Autodesk Inventor part; units mm, degrees
ref_plane "YZ Plane" through (0, 0, 0) normal (1, 0, 0) x (0, 1, 0)
ref_plane "XZ Plane" through (0, 0, 0) normal (0, 1, 0) x (-1, 0, 0)
ref_plane "XY Plane" through (0, 0, 0) normal (0, 0, 1) x (1, 0, 0)
sketch "Эскиз1" plane through (0, 0, 0) normal (0, 0, 1) x (1, 0, 0)
  line L0 (0, 0) -> (10, 0)
  line L1 (10, 0) -> (10, 10)
  line L2 (10, 10) -> (0, 10)
  line L3 (0, 10) -> (0, 0)
  dimension "d5" = 10
  dimension "d6" = 10
sketch "Эскиз2" plane through (0, 0, 0) normal (0, 1, 0) x (-1, 0, 0)
  line L0 (0, 0) -> (0, 200)
  line L1 (-50, 250) -> (-250, 250)
  arc A0 (0, 200) -> (-50, 250) centre (-50, 200) ccw
  point P0 (0, 250)
  dimension "d3" = 250
  dimension "d4" = 250
  dimension "d7" = 50
sweep "Сдвиг1" add profiles "Эскиз1" path "Эскиз2"
properties part number "4"
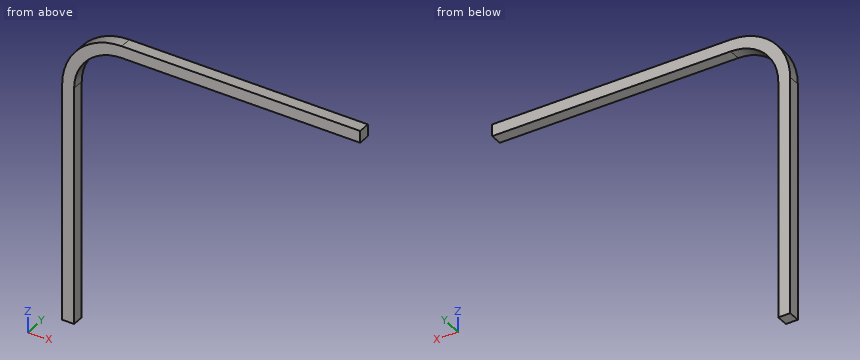
Here's how the part is built. I have some questions about the finished solid (model axes, mm). Round coordinates to 2 decimals unless told otherwise and drop trailing zeros. Write each loop counter-clockwise with the first axis right and the second up, starting at its lowest first coordinate (ties: lowest second). Pieces come first, ordered by that corner, then holes.
1. Suppose I cut it at C-C (x = 39.5). List the corners of the cut face in (y, z) for me, and give its area (3 significant figures).
2. Will these pins go through, and if not, where does the flat tip stop? pin 1 Ø3 at (y, z) = (4.5, 166.5) entering from +X; pin 2 Ø5 at (x, y) = (26, 7) entering from -Z.
3. Suppose I cut it at A-A (y = 3.75). List the corners of the cut face in (x, z) for me, and give its area (3 significant figures).
4. I need wall thicknesses on L1, parallel to X at y = 2.75, z = 76.5; L2, parallel to Z at x = 163, y = 3.5; L3, parallel to Z at x = 37.5, y = 3.25. Which ranges of each line are inside material? Lowest first, please.
5. Suppose I cut it at B-B (z = 149). List the corners of the cut face in (x, y) for me, and give its area (3 significant figures).
Answer sheet:
1. outline: (0, 238.6) - (10, 238.6) - (10, 248.89) - (0, 248.89) - close
1. area: 103 mm2
2. pin 1: stops at x = 10
2. pin 2: stops at z = 229.96
3. outline: (0, 0) - (10, 0) - (10, 200) arc R40 cw to (50, 240) - (250, 240) - (250, 250) - (50, 250) arc R50 ccw to (0, 200) - close
3. area: 4,710 mm2
4. L1: x = 0 to 10
4. L2: z = 240 to 250
4. L3: z = 238 to 248.41
5. outline: (0, 0) - (10, 0) - (10, 10) - (0, 10) - close
5. area: 100 mm2
